from build123d import *

# Parameters (mm, degrees)
SKETCH1_R             = 1
BOSS_EXTRUDE1_DEPTH   = 16
BOSS_EXTRUDE1_2_DEPTH = 16
BOSS_EXTRUDE2_DEPTH   = 16
SKETCH3_W             = 4.358106799
SKETCH3_H             = 21.361113411
BOSS_EXTRUDE4_DEPTH   = 1


with BuildPart() as part:
    # Sketch1 → Boss-Extrude1 (new body)
    with BuildSketch(Plane.XY):
        with Locations((-7.85, 0)):
            Circle(SKETCH1_R)
    extrude(amount=BOSS_EXTRUDE1_DEPTH)



with BuildPart() as body_2:
    # Sketch1 → Boss-Extrude1 2 (new body)
    with BuildSketch(Plane.XY):
        with Locations((7.85, 0)):
            Circle(SKETCH1_R)
    extrude(amount=BOSS_EXTRUDE1_2_DEPTH)


with BuildPart() as part_1:
    add(part.part)

    add(body_2.part)  # Boss-Extrude2 merges body 2
    # Sketch2 → Boss-Extrude2 (add, through all)
    with BuildSketch(Plane.XY):
        Polygon((7.85, 1), (10.7, 1), (10.7, -21.148770038), (-9.85, -21.148770038), (-9.85, 1), (-7.85, 1), (-7.85, -19.148770038), (8.7, -19.148770038), (8.7, -1.5), (7.85, -1.5), align=None)
    extrude(amount=BOSS_EXTRUDE2_DEPTH)

    # Sketch3 → Boss-Extrude4 (add)
    with BuildSketch(Plane.XY):
        with Locations((-7.670946601, -9.680556706)):
            Rectangle(SKETCH3_W, SKETCH3_H)
    extrude(amount=-BOSS_EXTRUDE4_DEPTH)


solid = part_1.part
Model file for the job. Use its own axes, mm. A direction names the side the tool comes from. Give positions to 0.01 mm unless a question says otherwise; leave off trailing zeros. Loops run counter-clockwise (first coordinate to the right, second up) from the corner with the lowest first, then second, coordinate; pieces in that order, holes last.
Item 1: Drop flat-ended pins along their axis: P1, Ø0.5, axis at x = -7.5, z = -0.5, coming from the -Y side; P2, Ø0.7, axis at x = -6, y = -10.5, coming from the +Z side. Give the stop position or say it passes through.
Check values:
P1: stops at y = -20.36
P2: stops at z = 0
Item 2: Slice it at C-C (y = -14). Write the cut outline in (x, z).
Check values:
outline: (-9.85, -1) - (-5.49, -1) - (-5.49, 0) - (-7.85, 0) - (-7.85, 16) - (-9.85, 16) - close; (8.7, 0) - (10.7, 0) - (10.7, 16) - (8.7, 16) - close
Item 3: Slice it at A-A (y = 0). Write the cut outline in (x, z).
Check values:
outline: (-9.85, -1) - (-5.49, -1) - (-5.49, 0) - (-6.85, 0) - (-6.85, 16) - (-9.85, 16) - close; (6.85, 0) - (10.7, 0) - (10.7, 16) - (6.85, 16) - close
Item 4: Slice it at B-B (z = 7). Write the cut outline in (x, y).
Check values:
outline: (-9.85, -21.15) - (10.7, -21.15) - (10.7, 1) - (7.85, 1) arc R1 ccw to (7.85, -1) - (7.85, -1.5) - (8.7, -1.5) - (8.7, -19.15) - (-7.85, -19.15) - (-7.85, -1) arc R1 ccw to (-7.85, 1) - (-9.85, 1) - close
Item 5: Slice it at D-D (x = 1.5). Write the cut outline in (y, z), plus the area to 3 significant figures.
Check values:
outline: (-21.15, 0) - (-19.15, 0) - (-19.15, 16) - (-21.15, 16) - close
area: 32.0 mm2
Item 6: Which spindle directions (+Z, -Z, +X, -X, +Y, -Y) get a long thin tool onto all of the face, cutting with end or side? Do faces 4 (the face through (-7.85, -10, 8)), 5 (the face through (9, 1, 8)), 6 (the face through (-7.7, -20.361, -0.5)), 7 (the face through (10.7, -10, 8)), 8 (the face through (8.7, -10, 8)). Say none if no direction does.
Check values:
face 4: +Z
face 5: +Z, -Z, +X, -X, +Y
face 6: -Z, +X, -X, -Y
face 7: +Z, -Z, +X, +Y, -Y
face 8: +Z, -Z
Item 7: Mould opens along X. For faces 1 (the face through (-5.492, -9.8, -0.5)), 2 (the face through (8, -1.5, 8)), 3 (the face through (-8, -10, -1)) say: +X half, -X half, draft (parallel to the pull), parting line (faces both ways), or undercut.
Check values:
face 1: +X half
face 2: undercut
face 3: draft
Item 8: Drill centre lines: line 1 along X through (y, z) = (-12, 14.5); line 2 along Y through (x, z) = (8.5, 8); line 3 along Y through (x, z) = (6, 14.75). Where is each one in solid material? Low to high.
Check values:
line 1: x = -9.85 to -7.85, 8.7 to 10.7
line 2: y = -21.15 to -19.15, -1.5 to 1
line 3: y = -21.15 to -19.15
